Work out the finished part from the listing and answer in its coordinate system (mm). Face numbers are marked on the shaded views. A direction names the side the tool comes from. Coordinates: 2 decimals unless noted, no trailing zeros. Order: outer loops, then holes, each group sorted by start corner. A loop starts at its lowest first (then second) coordinate and runs counter-clockwise, first axis right, second up. Notation, with made-up numbers: M 6.5,76 L 30.5,76 A18 cw 30.5,98 Z; hole C 6,-8.75 d11. An arc over 180 degrees is marked long. Write item = value, one per line. Start each with the question number.
Q1. Each of these flat-tipped pins is pushed along its axis until it touches: P1, Ø5.5, axis at x = 2.5, z = 1.5, coming from the +Y side; P2, Ø6, axis at y = 6, z = -16.5, coming from the -X side; P3, Ø1, axis at x = -4, z = -2.5, coming from the -Y side; P4, Ø10, axis at x = -9.5, z = -15.5, coming from the -Y side. Where does it stop, or does it pass through?
Q2. Find section A-A on y = 5.25. Give the vertices of the cut face in (x, z), and give its area (3 significant figures).
Q3. A tool of negligible diameter and unlimited length cuts with its end or side. For the marked faces 4 and 5, from which of +Z, -Z, +X, -X, +Y, -Y can it reach the whole face along a straight path? Write none if from no direction.
Q4. Straight lines are drawn through the part: line 1 along Y through (x, z) = (7.5, 16.5); line 2 along Z through (x, y) = (-3.25, 8.25); line 3 along Y through (x, z) = (-1.5, 6). For each, find the intervals that lie inside material, in ascending order.
Q5. Find section D-D on x = 0.5. Give the vertices of the cut face in (y, z).
Q6. Find section B-B on x = -10. Give the vertices of the cut face in (y, z), and give its area (3 significant figures).
Q7. Determine the mould class of the marked faces 1, 2 and 3 for opening direction Z: released by +Z, released by -Z, zero draft, split by the parting line, or undercut.
Q8. Find section C-C on z = 19. Give the vertices of the cut face in (x, y).
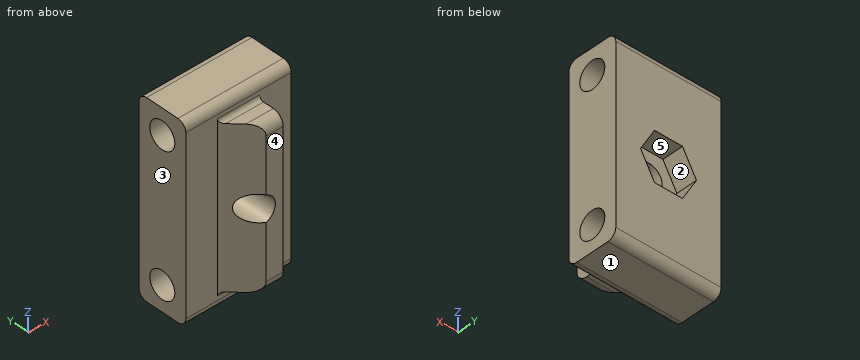
```python
from build123d import *

# Parameters (mm, degrees)
SKETCH1_W           = 25
SKETCH1_H           = 45
BOSS_EXTRUDE1_DEPTH = 12
CUT_EXTRUDE1_DEPTH  = 5
SKETCH3_R           = 3.15
CUT_EXTRUDE2_DEPTH  = 27.673957337
SKETCH8_R           = 3.2
CUT_EXTRUDE5_DEPTH  = 36.710642671
FILLET1_R           = 2
SKETCH10_W          = 10
SKETCH10_H          = 37.099879626
BOSS_EXTRUDE2_DEPTH = 6
CHAMFER1_SIZE       = 6
FILLET2_R           = 2.5
FILLET3_R           = 1
SKETCH12_R          = 3.15
CUT_EXTRUDE6_DEPTH  = 6


# Some blends are built 0.0001 mm under size
with BuildPart() as part:
    # Sketch1 → Boss-Extrude1 (new body)
    with BuildSketch(Plane(origin=(0, 0, 0), x_dir=(1, 0, 0), z_dir=(0, 1, 0))):
        Rectangle(SKETCH1_W, SKETCH1_H)
    extrude(amount=BOSS_EXTRUDE1_DEPTH)

    # Sketch2 → Cut-Extrude1 (cut)
    with BuildSketch(Plane(origin=(0, 12, 0), x_dir=(1, 0, 0), z_dir=(0, 1, 0))):
        Polygon((3.315, -5.741748427), (6.63, 0), (3.315, 5.741748427), (-3.315, 5.741748427), (-6.63, 0), (-3.315, -5.741748427), align=None)
    extrude(amount=-CUT_EXTRUDE1_DEPTH, mode=Mode.SUBTRACT)

    # Sketch3 → Cut-Extrude2 (cut, through all)
    with BuildSketch(Plane(origin=(0, 7, 0), x_dir=(1, 0, 0), z_dir=(0, 1, 0))):
        with Locations(Location((0, 0, 0), (0, 0, 270))):
            Circle(SKETCH3_R)
    extrude(amount=-CUT_EXTRUDE2_DEPTH, mode=Mode.SUBTRACT)

    # Sketch8 → Cut-Extrude5 (cut, through all)
    with BuildSketch(Plane.ZY.offset(12.5)):
        with Locations((16.5, 6)):
            Circle(SKETCH8_R)
    cut_extrude5 = extrude(amount=-CUT_EXTRUDE5_DEPTH, mode=Mode.SUBTRACT)

    # Mirror1: Cut-Extrude5 across plane
    add(cut_extrude5.mirror(Plane.XY), mode=Mode.SUBTRACT)

    # Fillet1
    fillet1_edges = [part.edges().sort_by_distance(p)[0] for p in [
        (0, 12, -22.5),
        (0, 0, -22.5),
        (0, 0, 22.5),
        (0, 12, 22.5),
    ]]
    fillet(fillet1_edges, radius=FILLET1_R)

    # Sketch10 → Boss-Extrude2 (add)
    with BuildSketch(Plane(origin=(0, 0, 0), x_dir=(-1, 0, 0), z_dir=(0, -1, 0))):
        Rectangle(SKETCH10_W, SKETCH10_H)
    extrude(amount=BOSS_EXTRUDE2_DEPTH)

    # Chamfer1
    chamfer1_edges = [part.edges().sort_by_distance(p)[0] for p in [
        (-5, -6, 0),
    ]]
    chamfer(chamfer1_edges, length=CHAMFER1_SIZE - 0.0001)  # a hair under: the kernel refuses the full size

    # Fillet2
    fillet2_edges = [part.edges().sort_by_distance(p)[0] for p in [
        (2.99995, -6, 18.549939813),
        (2.99995, -6, -18.549939813),
    ]]
    fillet(fillet2_edges, radius=FILLET2_R)

    # Fillet3
    # the kernel refuses this fillet: 1 mm, written as the material it adds along each edge
    with BuildSketch(Plane(origin=(-7.5, 0, -18.549939813), x_dir=(0, 0, -1), z_dir=(1, 0, 0))) as fillet3_piece_1_section:
        with BuildLine():
            CenterArc((FILLET3_R, -FILLET3_R), FILLET3_R, 90, 90)
            Line((0, -FILLET3_R), (0, 0))
            Line((0, 0), (FILLET3_R, 0))
        make_face()
    fillet3_piece_1 = extrude(amount=12.5, mode=Mode.PRIVATE)
    fillet3_piece_1 = split(fillet3_piece_1, bisect_by=Plane(origin=(-5.010050002, 0.009950002, -19.039939721), z_dir=(0.7071067811865476, 0.7071067811865476, 0)), keep=Keep.TOP, mode=Mode.PRIVATE)
    add(fillet3_piece_1)
    with BuildSketch(Plane(origin=(5, 0, 18.549939813), x_dir=(0, -1, 0), z_dir=(-1, 0, 0))) as fillet3_piece_2_section:
        with BuildLine():
            CenterArc((FILLET3_R, FILLET3_R), FILLET3_R, 180, 90)
            Line((0, FILLET3_R), (0, 0))
            Line((0, 0), (FILLET3_R, 0))
        make_face()
    fillet3_piece_2 = extrude(amount=12.5, mode=Mode.PRIVATE)
    fillet3_piece_2 = split(fillet3_piece_2, bisect_by=Plane(origin=(-2.333623853, -2.666476147, 18.779122608), z_dir=(0.7071067811865476, 0.7071067811865476, 0)), keep=Keep.TOP, mode=Mode.PRIVATE)
    add(fillet3_piece_2)

    # Sketch12 → Cut-Extrude6 (cut)
    with BuildSketch(Plane(origin=(0, 0, 0), x_dir=(1, 0, 0), z_dir=(0, 1, 0))):
        with Locations(Location((0, 0, 0), (0, 0, 270))):
            Circle(SKETCH12_R)
    extrude(amount=-CUT_EXTRUDE6_DEPTH, mode=Mode.SUBTRACT)


solid = part.part
```
Findings below:
q1.P1 = 7
q1.P2 = through
q1.P3 = -1.5
q1.P4 = -0.5
q2.outline = M -12.5,-22.5 L 12.5,-22.5 L 12.5,-19.61 L -12.5,-19.61 Z; M -12.5,-13.39 L 12.5,-13.39 L 12.5,13.39 L -12.5,13.39 Z; M -12.5,19.61 L 12.5,19.61 L 12.5,22.5 L -12.5,22.5 Z; hole C 0,0 d6.3
q2.area = 783 mm^2
q3.face_4 = +Z, -Z, +X, -X, -Y
q3.face_5 = +Y
q4.line_1 = 0 to 2.8, 9.2 to 12
q4.line_2 = -22.5 to -18.78, -14.22 to -5.74, 5.74 to 14.22, 18.78 to 22.5
q4.line_3 = -3.5 to 12
q5.outline = M -5.5,-17.55 A2.5 ccw -3.5,-18.55 L -1,-18.55 A1 cw 0,-19.55 L 0,-20.5 A2 ccw 2,-22.5 L 10,-22.5 A2 ccw 12,-20.5 L 12,-5.74 L 7,-5.74 L 7,-3.11 L -5.5,-3.11 Z; M -5.5,3.11 L 7,3.11 L 7,5.74 L 12,5.74 L 12,20.5 A2 ccw 10,22.5 L 2,22.5 A2 ccw 0,20.5 L 0,19.55 A1 cw -1,18.55 L -3.5,18.55 A2.5 ccw -5.5,17.55 Z; hole C 6,-16.5 d6.4; hole C 6,16.5 d6.4
q6.outline = M 0,-20.5 A2 ccw 2,-22.5 L 10,-22.5 A2 ccw 12,-20.5 L 12,20.5 A2 ccw 10,22.5 L 2,22.5 A2 ccw 0,20.5 Z; hole C 6,-16.5 d6.4; hole C 6,16.5 d6.4
q6.area = 472 mm^2
q7.face_1 = released by -Z
q7.face_2 = undercut
q7.face_3 = zero draft
q8.outline = M -12.5,0 L -5,0 L -4.84,-0.16 L 5,-0.16 L 5,0 L 12.5,0 L 12.5,4 L -12.5,4 Z; M -12.5,8 L 12.5,8 L 12.5,12 L -12.5,12 Z
